For this review, take the finished solid that the model builds, in its own axes (mm). Face numbers are marked on the shaded views. A direction names the side the tool comes from. Coordinates: 2 decimals unless noted, no trailing zeros. Write each loop counter-clockwise with the first axis right and the second up, starting at its lowest first coordinate (ties: lowest second). Pieces come first, ordered by that corner, then holes. Notation, with made-up numbers: M -35.75,33.5 L 11.25,33.5 A28 cw 11.25,66.5 Z; hole C -25,52 d10. An arc over 180 degrees is marked long. One line per question, with ' | ' between items.
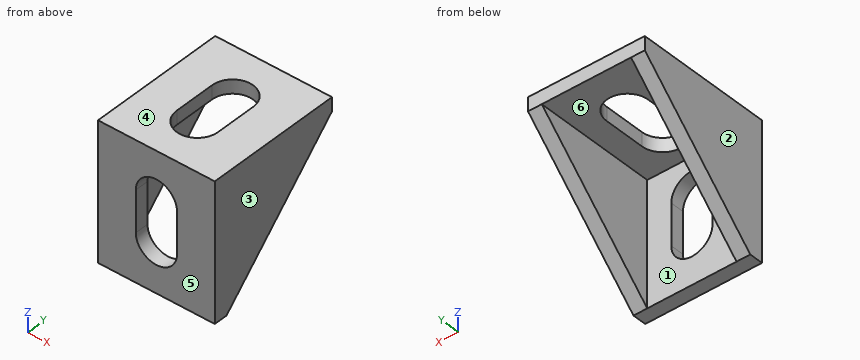
from build123d import *

# Parameters (mm, degrees)
BOSS_EXTRUDE1_DEPTH = 17
SKETCH2_W           = 13
SKETCH2_H           = 18
CUT_EXTRUDE1_DEPTH  = 18
CUT_EXTRUDE2_REACH  = 33.828
CUT_EXTRUDE3_REACH  = 33.828


with BuildPart() as part:
    # Sketch1 → Boss-Extrude1 (new body)
    with BuildSketch(Plane(origin=(0, 0, 0), x_dir=(0, 0, -1), z_dir=(1, 0, 0))):
        Polygon((0, 0), (0, 20), (2, 20), (20, 2), (20, 0), align=None)
    extrude(amount=BOSS_EXTRUDE1_DEPTH)

    # Sketch2 → Cut-Extrude1 (cut)
    with BuildSketch(Plane(origin=(0, 20, 0), x_dir=(1, 0, 0), z_dir=(0, 1, 0))):
        with Locations((8.5, 11)):
            Rectangle(SKETCH2_W, SKETCH2_H)
    extrude(amount=-CUT_EXTRUDE1_DEPTH, mode=Mode.SUBTRACT)

    # Sketch3 → Cut-Extrude2 (cut, up to next)
    with BuildSketch(Plane(origin=(0, 0, -2), x_dir=(-1, 0, 0), z_dir=(0, 0, -1)), mode=Mode.PRIVATE) as cut_extrude2_sk1:
        with BuildLine():
            Line((-11.5, 7), (-11.5, 13))
            ThreePointArc((-11.5, 13), (-8.5, 16), (-5.5, 13))
            Line((-5.5, 13), (-5.5, 7))
            ThreePointArc((-5.5, 7), (-8.5, 4), (-11.5, 7))
        make_face()
    cut_extrude2_tool1 = extrude(cut_extrude2_sk1.sketch, amount=-CUT_EXTRUDE2_REACH, mode=Mode.PRIVATE) & part.part
    add(cut_extrude2_tool1.solids().sort_by_distance((8.5, 10, -2))[0], mode=Mode.SUBTRACT)

    # Sketch4 → Cut-Extrude3 (cut, up to next)
    with BuildSketch(Plane(origin=(0, 2, 0), x_dir=(1, 0, 0), z_dir=(0, 1, 0)), mode=Mode.PRIVATE) as cut_extrude3_sk1:
        with BuildLine():
            Line((11.5, 13), (11.5, 7))
            ThreePointArc((11.5, 7), (8.5, 4), (5.5, 7))
            Line((5.5, 7), (5.5, 13))
            ThreePointArc((5.5, 13), (8.5, 16), (11.5, 13))
        make_face()
    cut_extrude3_tool1 = extrude(cut_extrude3_sk1.sketch, amount=-CUT_EXTRUDE3_REACH, mode=Mode.PRIVATE) & part.part
    add(cut_extrude3_tool1.solids().sort_by_distance((8.5, 2, -10))[0], mode=Mode.SUBTRACT)


solid = part.part
1) We need section D-D on z = -3. State the section outline as (x, y) points, then the cut area to 3 significant figures.
Responses:
outline: M 0,0 L 17,0 L 17,19 L 15,19 L 15,2 L 2,2 L 2,19 L 0,19 Z | area: 102 mm^2
2) We need section A-A on x = 8.5. State the section outline as (y, z) points, then the cut area to 3 significant figures.
Responses:
outline: M 0,-20 L 2,-20 L 2,-16 L 0,-16 Z; M 0,-4 L 2,-4 L 2,-2 L 4,-2 L 4,0 L 0,0 Z; M 16,-2 L 20,-2 L 20,0 L 16,0 Z | area: 28.0 mm^2
3) Insertion check: pin 1 Ø6.5 at (x, z) = (8, -12) entering from +Y; pin 2 Ø2 at (x, y) = (10.5, 16) entering from -Z. Each pin has a flat end and moves straight along its axis. Give the tip position at first contact, or say it passes through.
Responses:
pin 1: y = 2 | pin 2: z = -2
4) We need section B-B on z = -15.5. State the section outline as (x, y) points.
Responses:
outline: M 0,0 L 6.84,0 L 6.84,2 L 2,2 L 2,6.5 L 0,6.5 Z; M 10.16,0 L 17,0 L 17,6.5 L 15,6.5 L 15,2 L 10.16,2 Z
5) The part is to be moulded in two halves that separate along X. For the marked faces 1, 2, 3 and 4, say which applies: +X half, -X half, draft (parallel to the pull), parting line (faces both ways), or undercut.
Responses:
face 1: undercut | face 2: -X half | face 3: +X half | face 4: draft
6) Machinability: for the marked faces 5 and 6, which of the approach directions +Z, -Z, +X, -X, +Y, -Y give a long, thin tool a straight path to every point of the face, cutting with its end or side? Answer none if there is none.
Responses:
face 5: +Z, -Z, +X, -X, -Y | face 6: -Z, +Y
7) We need section C-C on y = 14.5. State the section outline as (x, z) points.
Responses:
outline: M 0,-7.5 L 2,-7.5 L 2,-2 L 5.9,-2 L 5.9,0 L 0,0 Z; M 11.1,-2 L 15,-2 L 15,-7.5 L 17,-7.5 L 17,0 L 11.1,0 Z
8) To check wall thickness, follow line 1 along X through (y, z) = (7.5, -2.25); line 2 along Z through (x, y) = (1.75, 9); line 3 along Y through (x, z) = (13.75, -6.25). State the ranges of each line that lie inside material, in increasing order. Write a range as [from, to].
Responses:
line 1: [0, 2], [15, 17] | line 2: [-13, 0] | line 3: [0, 2]
